Job drawing, mm, ordinate dimensions from the low corner. One solid piece. Coordinates: 2 decimals unless noted, no trailing zeros. Write each loop counter-clockwise with the first axis right and the second up, starting at its lowest first coordinate (ties: lowest second). Pieces come first, ordered by that corner, then holes. Notation, with made-up numbers: (83.25, 60) - (119.25, 60) arc R25 ccw to (119.25, 90) - close; hole circle Ø2 at (44, 46). An arc over 180 degrees is marked (long way). Put each result on its own line as item: value. Start each with the question number.
1. Drop flat-ended pins along their axis: P1, Ø12, axis at y = 12, z = 21.5, coming from the -X side; P2, Ø3, axis at y = 3.5, z = 20.5, coming from the -X side; P3, Ø12, axis at y = 3.5, z = 15, coming from the -X side. Give the stop position or say it passes through.
2. Saw through at A-A, the plane z = 65. Write the cut outline in (x, y), plus the area to 3 significant figures.
3. Saw through at B-B, the plane y = 2. Write the cut outline in (x, z), plus the area to 3 significant figures.
4. Pull direction Z, two halves, no side cores. Call the marked faces 1, 2, 3 and 4: released by +Z, released by -Z, zero draft, split by the parting line, or undercut.
5. Saw through at C-C, the plane x = 40. Write the cut outline in (y, z).
6. Drill centre lines: L1, parallel to X at y = 14.25, z = 65; L2, parallel to Z at x = 33.5, y = 1; L3, parallel to Z at x = 65, y = 6. Where is each one in solid material? Low to high. Write a range as from..to.
7. Saw through at D-D, the plane z = 36. Write the cut outline in (x, y).
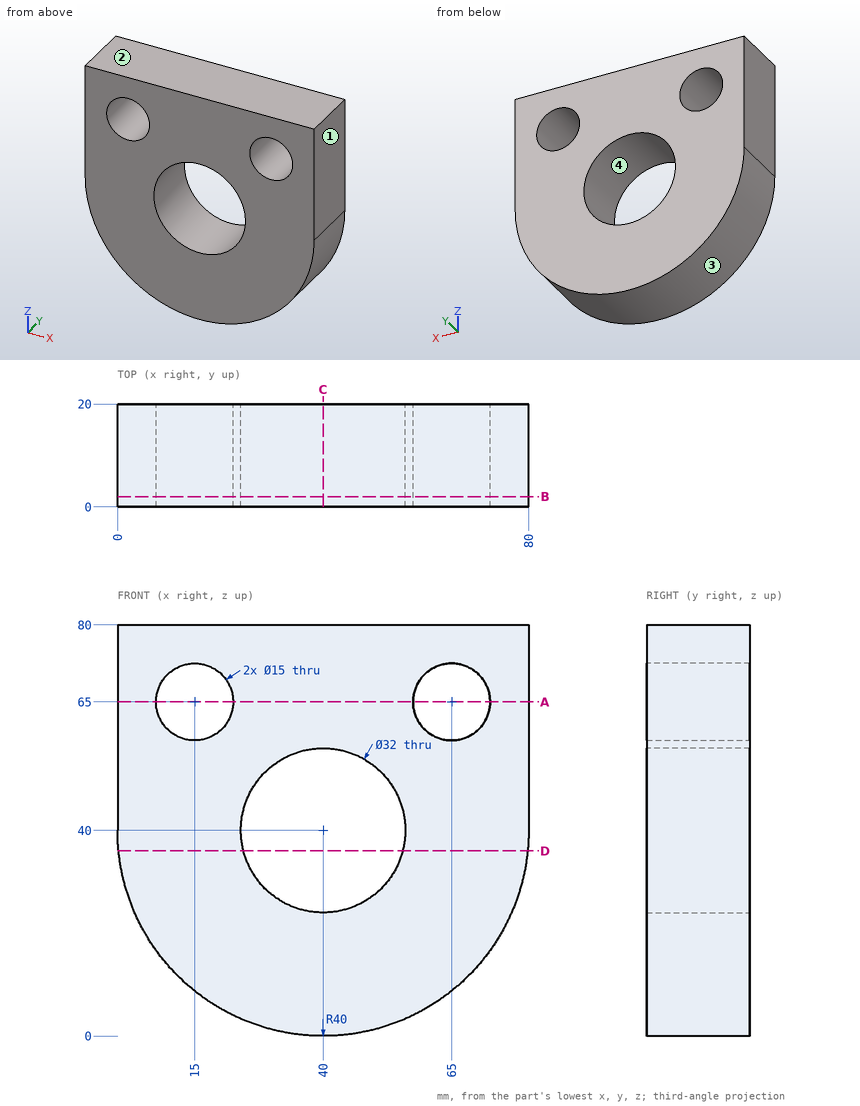
Final values:
1. P1: stops at x = 2
1. P2: stops at x = 4.28
1. P3: stops at x = 4.8
2. outline: (0, 0) - (7.5, 0) - (7.5, 20) - (0, 20) - close; (22.5, 0) - (57.5, 0) - (57.5, 20) - (22.5, 20) - close; (72.5, 0) - (80, 0) - (80, 20) - (72.5, 20) - close
2. area: 1,000 mm²
3. outline: (0, 40) arc R40 ccw to (80, 40) - (80, 80) - (0, 80) - close; hole circle Ø15 at (15, 65); hole circle Ø32 at (40, 40); hole circle Ø15 at (65, 65)
3. area: 4,560 mm²
4. face 1: zero draft
4. face 2: released by +Z
4. face 3: released by -Z
4. face 4: undercut
5. outline: (0, 0) - (20, 0) - (20, 24) - (0, 24) - close; (0, 56) - (20, 56) - (20, 80) - (0, 80) - close
6. L1: x = 0..7.5, 22.5..57.5, 72.5..80
6. L2: z = 0.53..25.38, 54.62..80
6. L3: z = 8.78..57.5, 72.5..80
7. outline: (0.2, 0) - (24.51, 0) - (24.51, 20) - (0.2, 20) - close; (55.49, 0) - (79.8, 0) - (79.8, 20) - (55.49, 20) - close
